Verification items for the finished model (mm, model axes). A direction names the side the tool comes from. Coordinates: 2 decimals unless noted, no trailing zeros. Write each loop counter-clockwise with the first axis right and the second up, starting at its lowest first coordinate (ties: lowest second). Pieces come first, ordered by that corner, then holes. Notation, with made-up numbers: (40.5, -5.75) -> (71.5, -5.75) arc R17 cw to (71.5, 14.25) -> close; hole circle Ø11 at (65.25, -3). An arc over 180 degrees is marked (long way). Answer in a Markdown table with one row per item.
```python
from build123d import *

# Parameters (mm, degrees)
SKETCH1_W           = 35
SKETCH1_H           = 60
SKETCH1_R           = 1
SKETCH1_W_2         = 22
SKETCH1_H_2         = 44
BOSS_EXTRUDE1_DEPTH = 5
SKETCH2_W           = 5
SKETCH2_H           = 50
BOSS_EXTRUDE2_DEPTH = 40
SKETCH3_R           = 1
CUT_EXTRUDE1_DEPTH  = 5


with BuildPart() as part:
    # Sketch1 → Boss-Extrude1 (new body)
    with BuildSketch(Plane.XY):
        with Locations((0, -1)):
            Rectangle(SKETCH1_W, SKETCH1_H)
        with Locations((-4.85, -24)):
            Circle(SKETCH1_R, mode=Mode.SUBTRACT)
        with Locations((4.85, -24)):
            Circle(SKETCH1_R, mode=Mode.SUBTRACT)
        with Locations((4.85, 24)):
            Circle(SKETCH1_R, mode=Mode.SUBTRACT)
        with Locations((-4.85, 24)):
            Circle(SKETCH1_R, mode=Mode.SUBTRACT)
        Rectangle(SKETCH1_W_2, SKETCH1_H_2, mode=Mode.SUBTRACT)
    extrude(amount=BOSS_EXTRUDE1_DEPTH)

    # Sketch2 → Boss-Extrude2 (add)
    with BuildSketch(Plane.XY):
        with Locations((-15, -56)):
            Rectangle(SKETCH2_W, SKETCH2_H)
    extrude(amount=BOSS_EXTRUDE2_DEPTH)

    # Sketch3 → Cut-Extrude1 (cut)
    with BuildSketch(Plane(origin=(-12.5, 0, 0), x_dir=(0, 0, -1), z_dir=(1, 0, 0))):
        with Locations(Location((-20, -74.5, 0), (0, 0, 90))):
            Circle(SKETCH3_R)
        with Locations(Location((-20, -71.5, 0), (0, 0, 90))):
            Circle(SKETCH3_R)
        with Locations(Location((-20, -68.5, 0), (0, 0, 90))):
            Circle(SKETCH3_R)
        with Locations(Location((-26.495190528, -64.75, 0), (0, 0, 90))):
            Circle(SKETCH3_R)
        with Locations(Location((-29.09326674, -66.25, 0), (0, 0, 90))):
            Circle(SKETCH3_R)
        with Locations(Location((-31.691342951, -67.75, 0), (0, 0, 90))):
            Circle(SKETCH3_R)
        with Locations(Location((-26.495190528, -57.25, 0), (0, 0, 90))):
            Circle(SKETCH3_R)
        with Locations(Location((-29.09326674, -55.75, 0), (0, 0, 90))):
            Circle(SKETCH3_R)
        with Locations(Location((-31.691342951, -54.25, 0), (0, 0, 90))):
            Circle(SKETCH3_R)
        with Locations(Location((-20, -53.5, 0), (0, 0, 90))):
            Circle(SKETCH3_R)
        with Locations(Location((-20, -50.5, 0), (0, 0, 90))):
            Circle(SKETCH3_R)
        with Locations(Location((-20, -47.5, 0), (0, 0, 90))):
            Circle(SKETCH3_R)
        with Locations(Location((-13.504809472, -57.25, 0), (0, 0, 90))):
            Circle(SKETCH3_R)
        with Locations(Location((-10.90673326, -55.75, 0), (0, 0, 90))):
            Circle(SKETCH3_R)
        with Locations(Location((-8.308657049, -54.25, 0), (0, 0, 90))):
            Circle(SKETCH3_R)
        with Locations(Location((-13.504809472, -64.75, 0), (0, 0, 90))):
            Circle(SKETCH3_R)
        with Locations(Location((-10.90673326, -66.25, 0), (0, 0, 90))):
            Circle(SKETCH3_R)
        with Locations(Location((-8.308657049, -67.75, 0), (0, 0, 90))):
            Circle(SKETCH3_R)
    extrude(amount=-CUT_EXTRUDE1_DEPTH, mode=Mode.SUBTRACT)


solid = part.part
```
1. Go/stop test with flat-tipped pins: pin 1 (12 mm diameter, centred on x = -9, z = 23, fed in from +Y); pin 2 (2.5 mm diameter, centred on y = -71.5, z = 20, fed in from +X); pin 3 (1.5 mm diameter, centred on x = 8.5, z = 2, fed in from -Y). Record where each tip stops, or that it passes through.
Findings below:
| item | result |
|---|---|
| pin 1 | stops at y = -31 |
| pin 2 | stops at x = -12.5 |
| pin 3 | stops at y = -31 |
2. Sectioned sample at B-B, the plane y = 4.5. Record the cut outline in (x, z), and give its area (3 significant figures).
Findings below:
| item | result |
|---|---|
| outline | (-17.5, 0) -> (-11, 0) -> (-11, 5) -> (-17.5, 5) -> close; (11, 0) -> (17.5, 0) -> (17.5, 5) -> (11, 5) -> close |
| area | 65.0 mm² |
3. Release check for a two-part mould opening along Y. For faces 3 (the face through (-17.5, -51, 15)), 4 (the face through (-14.96, -58.25, 13.55)), 5 (the face through (2, -31, 2)) record: released by +Y, released by -Y, zero draft, split by the parting line, or undercut.
Findings below:
| item | result |
|---|---|
| face 3 | zero draft |
| face 4 | undercut |
| face 5 | released by -Y |
4. Sectioned sample at C-C, the plane y = -36. Record the cut outline in (x, z), and give its area (3 significant figures).
Findings below:
| item | result |
|---|---|
| outline | (-17.5, 0) -> (-12.5, 0) -> (-12.5, 40) -> (-17.5, 40) -> close |
| area | 200 mm² |
5. Sectioned sample at D-D, the plane x = 13.5. Record the cut outline in (y, z).
Findings below:
| item | result |
|---|---|
| outline | (-31, 0) -> (29, 0) -> (29, 5) -> (-31, 5) -> close |
6. Access from +Z, -Z, +X, -X, +Y, -Y to the whole of each face (thin tool, end or side, straight path). Record for faces 1 (the face through (17.5, -1, 2)), 2 (the face through (0, -22, 2)).
Findings below:
| item | result |
|---|---|
| face 1 | +Z, -Z, +X, +Y, -Y |
| face 2 | +Z, -Z |
7. Sectioned sample at A-A, the plane x = 8.5. Record the cut outline in (y, z), and give its area (3 significant figures).
Findings below:
| item | result |
|---|---|
| outline | (-31, 0) -> (-22, 0) -> (-22, 5) -> (-31, 5) -> close; (22, 0) -> (29, 0) -> (29, 5) -> (22, 5) -> close |
| area | 80.0 mm² |
8. Material ranges on probe 1 along Z at (x, y) = (-15.4, -64.75); probe 2 along Y at (x, z) = (4.85, 3.1); probe 3 along Y at (x, z) = (-14.5, 26.5), recorded low to high. Write a range as from..to.
Findings below:
| item | result |
|---|---|
| probe 1 | z = 0..12.5, 14.5..25.5, 27.5..40 |
| probe 2 | y = -31..-25, -23..-22, 22..23, 25..29 |
| probe 3 | y = -81..-65.75, -63.75..-58.25, -56.25..-31 |
